Source: CAD feature listing. Evaluate the final solid. Frame: model axes, mm. Face numbers are marked on the shaded views. A direction names the side the tool comes from. Coordinates: 2 decimals unless noted, no trailing zeros. Write each loop counter-clockwise with the first axis right and the second up, starting at its lowest first coordinate (ties: lowest second). Pieces come first, ordered by that corner, then holes. Notation, with made-up numbers: (-15.5, 73) -> (30.5, 73) arc R17 ccw to (30.5, 105) -> close; hole circle Ø7 at (-5.5, -38). An arc over 180 degrees is marked (long way). One line per item, written item: value. Start each with the question number.
1. Access query for the marked faces 1, 2 and 3. Directions: +Z, -Z, +X, -X, +Y, -Y. A direction counts if a zero-diameter tool reaches every point of the face in a straight line with its end or side. Return the directions, or none.
2. Section query C-C, the plane x = 77.5. Output: boundary loops of the cut face in (y, z).
3. Line query: line 1 (Y direction, x = 51, z = 22); line 2 (Z direction, x = 15, y = 53.75); line 3 (X direction, y = 11, z = 30). Output: solid intervals per line, ascending.
4. Section query B-B, the plane z = 19. Output: boundary loops of the cut face in (x, y), and give its area (3 significant figures).
5. First-contact query: P1, Ø18, axis at x = 15, z = 25, coming from the +Y side; P2, Ø1.5, axis at y = 1.5, z = 21, coming from the +X side; P3, Ø5.5, axis at x = 70.5, y = 57.5, coming from the +Z side; P4, Ø3, axis at x = 21, y = 46, coming from the +Z side. Flat tips, straight axial feed; report the tip coordinate or a pass-through.
6. Mould query, pull axis Z, two halves, no side actions, for the marked faces 4, 5 and 6. Classes: released by +Z, released by -Z, zero draft, split by the parting line, or undercut.
7. Section query D-D, the plane y = 9. Output: boundary loops of the cut face in (x, z).
8. Section query A-A, the plane x = 15. Output: boundary loops of the cut face in (y, z).
from build123d import *

# Parameters (mm, degrees)
SKETCH_W               = 90
SKETCH_H               = 60
PAD_DEPTH              = 10
PAD001_DEPTH           = 7.5
PAD002_DEPTH           = 2.5
LINEARPATTERN_COUNT    = 2
LINEARPATTERN_PITCH    = 45
LINEARPATTERN001_COUNT = 2
LINEARPATTERN001_PITCH = 45
SKETCH003_R            = 10
POCKET_DEPTH           = 60


with BuildPart() as part:
    # Sketch → Pad (new body)
    with BuildSketch(Plane.XY):
        with Locations((45, 30)):
            Rectangle(SKETCH_W, SKETCH_H)
    extrude(amount=PAD_DEPTH)

    # Sketch001 → Pad001 (join, symmetric)
    with BuildSketch(Plane.XZ.offset(-7.5)):
        with BuildLine():
            Line((0, 25), (0, 10))
            Line((0, 10), (30, 10))
            Line((30, 10), (30, 25))
            ThreePointArc((30, 25), (15, 40.000025), (0, 25))
        make_face()
    pad001 = extrude(amount=PAD001_DEPTH, both=True)

    # Sketch002 → Pad002 (join, symmetric)
    with BuildSketch(Plane.XZ.offset(-7.5)):
        with BuildLine():
            Line((30, 25), (30, 10))
            Line((30, 10), (90, 10))
            Line((20.769255, 38.846169), (90, 10))
            ThreePointArc((30, 25), (27.480768, 33.320507), (20.769255, 38.846169))
        make_face()
    pad002 = extrude(amount=PAD002_DEPTH, both=True)

    # LinearPattern: Pad001 ×2
    with Locations(*[(0, i * LINEARPATTERN_PITCH, 0) for i in range(1, LINEARPATTERN_COUNT)]):
        add(pad001)

    # LinearPattern001: Pad002 ×2
    with Locations(*[(0, i * LINEARPATTERN001_PITCH, 0) for i in range(1, LINEARPATTERN001_COUNT)]):
        add(pad002)

    # Sketch003 (on Face5 of LinearPattern001) → Pocket (cut)
    with BuildSketch(Plane.XZ):
        with Locations((15, 25.000025)):
            Circle(SKETCH003_R)
    extrude(amount=-POCKET_DEPTH, mode=Mode.SUBTRACT)


solid = part.part
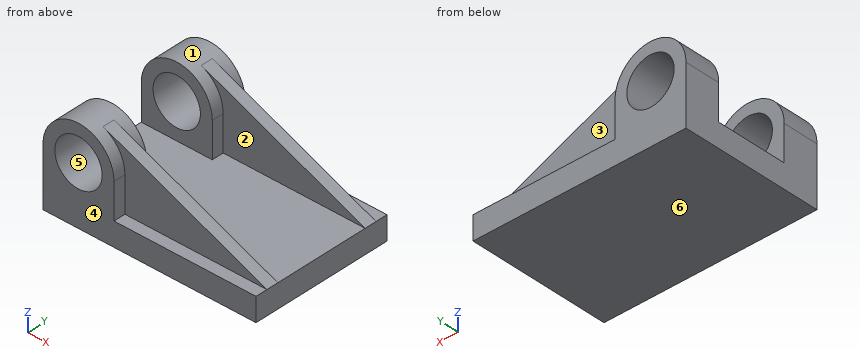
Computed values:
1. face 1: +Z
1. face 2: +Z, +X
1. face 3: +Z, +X, +Y
2. outline: (0, 0) -> (60, 0) -> (60, 10) -> (55, 10) -> (55, 15.21) -> (50, 15.21) -> (50, 10) -> (10, 10) -> (10, 15.21) -> (5, 15.21) -> (5, 10) -> (0, 10) -> close
3. line 1: y = 5 to 10, 50 to 55
3. line 2: z = 0 to 15, 35 to 40
3. line 3: x = 0.86 to 6.34, 23.66 to 29.14
4. outline: (0, 0) -> (7, 0) -> (7, 15) -> (0, 15) -> close; (0, 45) -> (7, 45) -> (7, 60) -> (0, 60) -> close; (23, 0) -> (30, 0) -> (30, 5) -> (68.4, 5) -> (68.4, 10) -> (30, 10) -> (30, 15) -> (23, 15) -> close; (23, 45) -> (30, 45) -> (30, 50) -> (68.4, 50) -> (68.4, 55) -> (30, 55) -> (30, 60) -> (23, 60) -> close
4. area: 804 mm²
5. P1: passes through
5. P2: stops at x = 30
5. P3: stops at z = 18.6
5. P4: stops at z = 39.31
6. face 4: zero draft
6. face 5: undercut
6. face 6: released by -Z
7. outline: (0, 0) -> (90, 0) -> (90, 10) -> (20.77, 38.85) arc R15 ccw to (0, 25) -> close; hole circle Ø20 at (15, 25)
8. outline: (0, 0) -> (60, 0) -> (60, 15) -> (45, 15) -> (45, 10) -> (15, 10) -> (15, 15) -> (0, 15) -> close; (0, 35) -> (15, 35) -> (15, 40) -> (0, 40) -> close; (45, 35) -> (60, 35) -> (60, 40) -> (45, 40) -> close
